```python
from build123d import *

# Parameters (mm, degrees)
SKETCH1_R             = 9.5
SKETCH1_R_2           = 3.96875
BOSS_EXTRUDE1_DEPTH   = 6.35
F_3_0MM_DOWEL_HOLE1_D = 3
CIRPATTERN1_COUNT     = 4
FILLET1_R             = 0.5


with BuildPart() as part:
    # Sketch1 → Boss-Extrude1 (new body)
    with BuildSketch(Plane.XY):
        Circle(SKETCH1_R)
        Circle(SKETCH1_R_2, mode=Mode.SUBTRACT)
    extrude(amount=BOSS_EXTRUDE1_DEPTH)

    # Ø3.0mm Dowel Hole1 (through all)
    with Locations(Plane.XY.offset(6.35)):
        with Locations((0, 8.89)):
            f_3_0mm_dowel_hole1 = Hole(F_3_0MM_DOWEL_HOLE1_D / 2)

    # CirPattern1: Ø3.0mm Dowel Hole1 ×4 about axis
    cirpattern1_axis = Axis((0, 0, 0), (0, 0, 1))
    for i in range(1, CIRPATTERN1_COUNT):
        add(f_3_0mm_dowel_hole1.rotate(cirpattern1_axis, i * 360 / CIRPATTERN1_COUNT), mode=Mode.SUBTRACT)

    # Fillet1
    fillet1_edges = [part.edges().sort_by_distance(p)[0] for p in [
        (-1.412656886, 9.394381327, 3.175),
        (1.412656886, 9.394381327, 3.175),
        (-9.394381327, -1.412656886, 3.175),
        (-9.394381327, 1.412656886, 3.175),
        (1.412656886, -9.394381327, 3.175),
        (-1.412656886, -9.394381327, 3.175),
        (9.394381327, 1.412656886, 3.175),
        (9.394381327, -1.412656886, 3.175),
    ]]
    fillet(fillet1_edges, radius=FILLET1_R)


solid = part.part
```
Build history of the part. All positions in model axes, mm. Give positions to 0.01 mm unless a question says otherwise; leave off trailing zeros. Order: outer loops, then holes, each group sorted by start corner. A loop starts at its lowest first (then second) coordinate and runs counter-clockwise, first axis right, second up. Notation, with made-up numbers: M 31.5,-14.5 L 71.5,-14.5 A32 cw 71.5,19.5 Z; hole C 42.5,45 d11. An arc over 180 degrees is marked long. Write item = value, one per line. Start each with the question number.
(1) Slice it at C-C on x = 5.5. Write the cut outline in (y, z), plus the area to 3 significant figures.
(2) Two-plate mould, pull along Y, no slides. Class faces 1 (the cylindrical face through (6.77, 6.664, 3.131)), 2 (the cylindrical face through (-0.86, -3.874, 3.131)), 3 (the flat face through (-4.3, 0.1, 6.35)), 4 (the cylindrical face through (6.664, -6.77, 3.131)): released by +Y, released by -Y, zero draft, split by the parting line, or undercut.
(3) Slice it at D-D on x = -4.75. Write the cut outline in (y, z), plus the area to 3 significant figures.
(4) Pin check, flat tip, straight feed: pin 1 Ø7 at (x, y) = (0, 0) entering from +Z. Stop position of the tip, or through.
(5) Slice it at A-A on x = 0. Write the cut outline in (y, z).
(6) Probe L1, parallel to Y at x = 0, z = 3.25; L2, parallel to Y at x = 2, z = 3.75; L3, parallel to X at y = -3.25, z = 1. List the from-to ranges inside material, lowest first. Write a range as [from, to].
Responses:
q1.outline = M -7.75,0 L 7.75,0 L 7.75,6.35 L -7.75,6.35 Z
q1.area = 98.4 mm2
q2.face_1 = released by +Y
q2.face_2 = undercut
q2.face_3 = zero draft
q2.face_4 = released by -Y
q3.outline = M -8.23,0 L 8.23,0 L 8.23,6.35 L -8.23,6.35 Z
q3.area = 104 mm2
q4.pin_1 = through
q5.outline = M -7.39,0 L -3.97,0 L -3.97,6.35 L -7.39,6.35 Z; M 3.97,0 L 7.39,0 L 7.39,6.35 L 3.97,6.35 Z
q6.L1 = [-7.39, -3.97], [3.97, 7.39]
q6.L2 = [-9.28, -3.43], [3.43, 9.28]
q6.L3 = [-8.93, -2.28], [2.28, 8.93]
